```python
from build123d import *

# Parameters (mm, degrees)
SKETCH_2_R      = 1.06
EXTRUDE_1_DEPTH = 0.75
FILLET_1_R      = 2.65
FILLET_2_R      = 1.59


with BuildPart() as part:
    # 草图2 → 拉伸1 (new, symmetric)
    with BuildSketch(Plane.XY):
        with BuildLine():
            Line((5.730721037, 19.810931144), (8.300141741, 24.087165303))
            Line((8.300141741, 24.087165303), (10.818460752, 28.278351963))
            ThreePointArc((10.818460752, 28.278351963), (0, 30.277124745), (-10.818460752, 28.278351963))
            Line((-10.818460752, 28.278351963), (-5.730721037, 19.810931144))
            ThreePointArc((-5.730721037, 19.810931144), (0, 20.623146132), (5.730721037, 19.810931144))
        make_face()
        with Locations((-4.7625, 25.477124745)):
            Circle(SKETCH_2_R, mode=Mode.SUBTRACT)
        with Locations((4.7625, 25.477124745)):
            Circle(SKETCH_2_R, mode=Mode.SUBTRACT)
    extrude(amount=EXTRUDE_1_DEPTH, both=True)

    # 圆角1
    fillet_1_edges = [part.edges().sort_by_distance(p)[0] for p in [
        (-10.818460752, 28.278351963, 0),
        (10.818460752, 28.278351963, 0),
    ]]
    fillet(fillet_1_edges, radius=FILLET_1_R)

    # 圆角2
    fillet_2_edges = [part.edges().sort_by_distance(p)[0] for p in [
        (-5.730721037, 19.810931144, 0),
        (5.730721037, 19.810931144, 0),
    ]]
    fillet(fillet_2_edges, radius=FILLET_2_R)


solid = part.part
```
For this review, take the finished solid that the model builds, in its own axes (mm). Give positions to 0.01 mm unless a question says otherwise; leave off trailing zeros. Loops run counter-clockwise (first coordinate to the right, second up) from the corner with the lowest first, then second, coordinate; pieces in that order, holes last. Notation, with made-up numbers: M 19.5,23 L 36.5,23 A19 ccw 36.5,40 Z; hole C 0.25,36 d5. An arc over 180 degrees is marked long. One line per item, written item: value. Start each with the question number.
Q1. Add section C-C (x = 0.75). Give the boundary of the cut face in (y, z), and give its area (3 significant figures).
Q2. Draft analysis for pull direction X (two halves, no side actions). For faces 1 (the face through (-7.737, 23.15, 0.01)), 2 (the face through (0.106, 30.277, 0.01)), 3 (the face through (4.533, 24.442, -0.01)), state which applies: released by +X, released by -X, zero draft, split by the parting line, or undercut.
Q3. Add section A-A (z = -0.45). Give the boundary of the cut face in (x, y).
Q4. Add section B-B (y = 23.5). Give the boundary of the cut face in (x, z).
Q5. For L1, parallel to X at y = 25, z = 0.2; L2, parallel to X at y = 26, z = -0.6; L3, parallel to Y at x = -4, z = 0.05, list the stretches that pass through material, from the lowest coordinate up.
Reply:
1. outline: M 20.61,-0.75 L 30.27,-0.75 L 30.27,0.75 L 20.61,0.75 Z
1. area: 14.5 mm²
2. face 1: released by -X
2. face 2: split by the parting line
2. face 3: undercut
3. outline: M -9.09,25.41 L -6.34,20.83 A1.59 ccw -4.62,20.1 A20.62 cw 4.62,20.1 A1.59 ccw 6.34,20.83 L 9.09,25.41 A2.65 ccw 7.48,29.34 A30.28 ccw -7.48,29.34 A2.65 ccw Z; hole C -4.76,25.48 d2.12; hole C 4.76,25.48 d2.12
4. outline: M -7.95,-0.75 L 7.95,-0.75 L 7.95,0.75 L -7.95,0.75 Z
5. L1: -8.85 to -5.71, -3.82 to 3.82, 5.71 to 8.85
5. L2: -9.36 to -5.68, -3.84 to 3.84, 5.68 to 9.36
5. L3: 20.23 to 24.74, 26.21 to 30.01
